Autodesk Inventor part; units mm, degrees
ref_plane "YZ Plane" through (0, 0, 0) normal (1, 0, 0) x (0, 1, 0)
ref_plane "XZ Plane" through (0, 0, 0) normal (0, 1, 0) x (-1, 0, 0)
ref_plane "XY Plane" through (0, 0, 0) normal (0, 0, 1) x (1, 0, 0)
sketch "Эскиз1" plane through (0, 0, 0) normal (0, 0, 1) x (1, 0, 0)
  circle A0 centre (0, 0) radius 90
  dimension "d0" = 180
extrude "Выдавливание1" add sketch "Эскиз1" along normal blind 8
sketch "Эскиз2" plane through (0, 0, 8) normal (0, 0, 1) x (1, 0, 0)
  point P0 (0, 0)
sketch "Эскиз3" plane through (0, 0, 8) normal (0, 0, 1) x (1, 0, 0)
  circle A0 centre (0, 0) radius 70
  dimension "d4" = 140
extrude "Выдавливание2" add sketch "Эскиз3" along normal blind 65
sketch "Эскиз4" plane through (0, 0, 0) normal (0, 0, -1) x (-1, 0, 0)
  circle A0 centre (0, 0) radius 65
  dimension "d7" = 130
extrude "Выдавливание3" cut sketch "Эскиз4" against normal blind 63
chamfer "Фаска1" distance 1 angle 45 1 edges at (65, 0, 0)
chamfer "Фаска2" distance 2 angle 45 1 edges at (-70, 0, 73)
sketch "Эскиз5" plane through (0, 0, 8) normal (0, 0, 1) x (1, 0, 0)
  line L0 (0, 0) -> (0, 90)
  circle A0 centre (0, 0) radius 90
  line L1 (0, 0) -> (-77.9423, 45)
  line L2 (0, 0) -> (-77.9423, -45)
  line L3 (0, 0) -> (0, -90)
  line L4 (0, 0) -> (77.9423, -45)
  line L5 (0, 0) -> (77.9423, 45)
  dimension "d18" = 360
sketch "Эскиз6" plane through (0, 0, 8) normal (0, 0, 1) x (1, 0, 0)
  point P0 (0, 0)
sketch "Эскиз7" plane through (0, 0, 8) normal (0, 0, 1) x (1, 0, 0)
  point P0 (0, 0)
sketch "Эскиз8" plane through (0, 0, 8) normal (0, 0, 1) x (1, 0, 0)
  point P0 (0, 0)
sketch "Эскиз9" plane through (0, 0, 73) normal (0, 0, 1) x (1, 0, 0)
  point P0 (0, 0)
sketch "Эскиз10" plane through (0, 0, 73) normal (0, 0, 1) x (1, 0, 0)
  circle A0 centre (0, 0) radius 57.5
  dimension "d20" = 115
sketch "Эскиз11" plane through (0, 0, 63) normal (0, 0, -1) x (-1, 0, 0)
  circle A0 centre (0, 0) radius 57.5
  dimension "d21" = 115
hole "Отверстие1" at (0, 0, 73) direction (0, 0, -1) diameter 115 end through all
sketch "Эскиз12" plane through (0, 0, 8) normal (0, 0, 1) x (1, 0, 0)
  circle A0 centre (0, 0) radius 80
  circle A1 centre (0, 0) radius 70
  point P0 (0, 80)
  point P1 (-69.282, 40)
  point P2 (-69.282, -40)
  point P3 (0, -80)
  point P4 (69.282, -40)
  point P5 (69.282, 40)
  dimension "d29" = 160
  dimension "d32" = 360
hole "Отверстие2" at (0, 80, 8) at (69.282, 40, 8) at (69.282, -40, 8) at (0, -80, 8) at (-69.282, -40, 8) at (-69.282, 40, 8) direction (0, 0, -1) diameter 11 end through all
fillet "Сопряжение1" radius 0.6 1 edges at (-70, 0, 8)
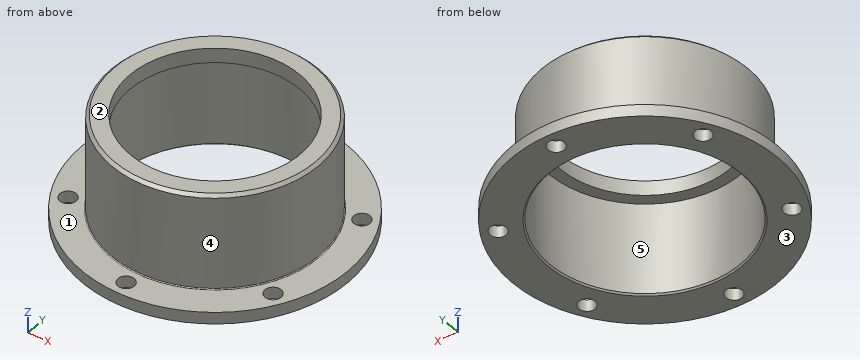
Check sheet for the modelled part. Datum: model origin and axes. Units: mm. Face numbers are marked on the shaded views. A direction names the side the tool comes from. Coordinates: 2 decimals unless noted, no trailing zeros. Write each loop counter-clockwise with the first axis right and the second up, starting at its lowest first coordinate (ties: lowest second). Pieces come first, ordered by that corner, then holes. Notation, with made-up numbers: M 45.5,40.5 L 51.5,40.5 A19 cw 51.5,63.5 Z; hole C 68,61.25 d2. An arc over 180 degrees is marked long. Answer as CSV lines item,"result".
Q1. Set-up check for the marked faces 1 and 2: record each of +Z, -Z, +X, -X, +Y, -Y from which the full face is reachable in a straight line by a thin tool's end or side.
Check result:
face 1,"+Z"
face 2,"+Z, +X, -X, +Y, -Y"
Q2. Cross-section at B-B (x = 0). Count the separate pieces of the cut face and the enclosed holes in it, then the cut area to 3 significant figures.
Check result:
separate pieces,"4"
enclosed holes,"0"
area,"1,020 mm^2"
Q3. Mould release check, pull along Y, two halves, no side actions. Record for the marked faces 3, 4 and 5: released by +Y, released by -Y, zero draft, split by the parting line, or undercut.
Check result:
face 3,"zero draft"
face 4,"split by the parting line"
face 5,"undercut"
Q4. Go/stop test with flat-tipped pins: pin 1 (3 mm diameter, centred on y = 23, z = 57.5, fed in from -X); pin 2 (14.5 mm diameter, centred on x = -69.282, y = 40, fed in from +Z); pin 3 (2 mm diameter, centred on y = 55, z = 31.5, fed in from +X). Record where each tip stops, or that it passes through.
Check result:
pin 1,"x = -66.62"
pin 2,"z = 8"
pin 3,"x = 44.54"
Q5. Cross-section at A-A (y = 0). Record the boundary of the cut face in (x, z).
Check result:
outline,"M -90,0 L -66,0 L -65,1 L -65,63 L -57.5,63 L -57.5,73 L -68,73 L -70,71 L -70,8.6 A0.6 cw -70.6,8 L -90,8 Z; M 57.5,63 L 65,63 L 65,1 L 66,0 L 90,0 L 90,8 L 70.6,8 A0.6 cw 70,8.6 L 70,71 L 68,73 L 57.5,73 Z"
Q6. Cross-section at C-C (z = 57). Record the boundary of the cut face in (x, y), then the cut area to 3 significant figures.
Check result:
outline,"C 0,0 d140; hole C 0,0 d130"
area,"2,120 mm^2"
Q7. Material ranges on probe 1 along Y at (x, z) = (0, 6.25); probe 2 along Y at (x, z) = (0, 66); probe 3 along Y at (x, z) = (35.5, 55), recorded low to high. Write a range as from..to.
Check result:
probe 1,"-90..-85.5, -74.5..-65, 65..74.5, 85.5..90"
probe 2,"-70..-57.5, 57.5..70"
probe 3,"-60.33..-54.45, 54.45..60.33"
Q8. Cross-section at D-D (y = 80). Record the boundary of the cut face in (x, z).
Check result:
outline,"M -41.23,0 L -5.5,0 L -5.5,8 L -41.23,8 Z; M 5.5,0 L 41.23,0 L 41.23,8 L 5.5,8 Z"
